```python
from build123d import *

# Parameters (mm, degrees)
SKETCH1_R           = 1.5
BOSS_EXTRUDE1_DEPTH = 38
SKETCH2_R           = 3
BOSS_EXTRUDE2_DEPTH = 8
BOSS_EXTRUDE3_START = -50
SKETCH2_2_R         = 3
BOSS_EXTRUDE3_DEPTH = 8
CHAMFER1_SIZE       = 0.5
SKETCH3_R           = 5
BOSS_EXTRUDE4_DEPTH = 8
CUT_EXTRUDE1_DEPTH  = 8
SKETCH5_R           = 2
CUT_EXTRUDE2_DEPTH  = 47.957427527
CHAMFER3_SIZE       = 1
FILLET1_R           = 2
CHAMFER4_SIZE       = 1


with BuildPart() as part:
    # Sketch1 → Boss-Extrude1 (new, symmetric)
    with BuildSketch(Plane(origin=(0, 0, 0), x_dir=(0, 0, -1), z_dir=(1, 0, 0))):
        Circle(SKETCH1_R)
    extrude(amount=BOSS_EXTRUDE1_DEPTH, both=True)

    # Sketch2 → Boss-Extrude2 (add)
    with BuildSketch(Plane(origin=(38, 0, 0), x_dir=(0, 0, -1), z_dir=(1, 0, 0))):
        Circle(SKETCH2_R)
    extrude(amount=BOSS_EXTRUDE2_DEPTH)

    # Sketch2<2> → Boss-Extrude3 (add)
    with BuildSketch(Plane(origin=(38, 0, 0), x_dir=(0, 0, -1), z_dir=(1, 0, 0)).offset(BOSS_EXTRUDE3_START)):
        Circle(SKETCH2_2_R)
    extrude(amount=BOSS_EXTRUDE3_DEPTH)

    # Chamfer1
    chamfer1_edges = [part.edges().sort_by_distance(p)[0] for p in [
        (-12, 0, 3),
        (-4, 0, 3),
        (38, 0, 3),
        (46, 0, 3),
    ]]
    chamfer(chamfer1_edges, length=CHAMFER1_SIZE)

    # Sketch3 → Boss-Extrude4 (add)
    with BuildSketch(Plane.ZY.offset(38)):
        Circle(SKETCH3_R)
    extrude(amount=-BOSS_EXTRUDE4_DEPTH)

    # Sketch4 → Cut-Extrude1 (cut)
    with BuildSketch(Plane.ZY.offset(38)):
        with BuildLine():
            Line((-4, 3), (-4, -3))
            ThreePointArc((-4, -3), (-5, 0), (-4, 3))
        make_face()
        with BuildLine():
            Line((4, 3), (4, -3))
            ThreePointArc((4, -3), (5, 0), (4, 3))
        make_face()
    extrude(amount=-CUT_EXTRUDE1_DEPTH, mode=Mode.SUBTRACT)

    # Sketch5 → Cut-Extrude2 (cut, through all)
    with BuildSketch(Plane.XY.offset(4)):
        with Locations((-34, 0)):
            Circle(SKETCH5_R)
    extrude(amount=-CUT_EXTRUDE2_DEPTH, mode=Mode.SUBTRACT)

    # Chamfer3
    chamfer3_edges = [part.edges().sort_by_distance(p)[0] for p in [
        (-38, 5, 0),
        (-38, -5, 0),
    ]]
    chamfer(chamfer3_edges, length=CHAMFER3_SIZE - 0.0001)  # a hair under: the kernel refuses the full size

    # Fillet1
    fillet1_edges = [part.edges().sort_by_distance(p)[0] for p in [
        (-30, 0, 1.5),
    ]]
    fillet(fillet1_edges, radius=FILLET1_R)

    # Chamfer4
    chamfer4_edges = [part.edges().sort_by_distance(p)[0] for p in [
        (-30, 5, 0),
        (-30, -5, 0),
    ]]
    chamfer(chamfer4_edges, length=CHAMFER4_SIZE - 0.0001)  # a hair under: the kernel refuses the full size


solid = part.part
```
Geometry: final body of the model. Coordinates: model frame, mm. A direction names the side the tool comes from. Round coordinates to 2 decimals unless told otherwise and drop trailing zeros. Order: outer loops, then holes, each group sorted by start corner. A loop starts at its lowest first (then second) coordinate and runs counter-clockwise, first axis right, second up. Notation, with made-up numbers: (33, 44) -> (38, 44) arc R29 ccw to (38, 74) -> close; hole circle Ø9 at (-8, 30). An arc over 180 degrees is marked (long way). Use one line per item in the form item = value. Start each with the question number.
1. Cut plane C-C (x = 25.5). Return the cut outline in (y, z), then the cut area to 3 significant figures.
2. Cut plane A-A (x = -34). Return the cut outline in (y, z), then the cut area to 3 significant figures.
3. Reachability of faces 4 (the face through (-19.89, 0.07, 1.5)), 5 (the face through (-8, 0, 3)), 6 (the face through (46, 0, 0)) from +Z, -Z, +X, -X, +Y, -Y: full face, straight path, thin tool, end or side. Return the list, or none.
4. Line query: probe 1 along Y at (x, z) = (-34, 1.75); probe 2 along Y at (x, z) = (-34, 2); probe 3 along X at (y, z) = (-2.5, 2.25). Output: solid intervals per line, ascending.
5. Draft query along X for faces 1 (the face through (-30.2, 4.2, 0.1)), 2 (the face through (-34, -5, 0)), 3 (the face through (38, -2, 0)). Return one class per face: pulls with the +X half, pulls with the -X half, needs draft (parallel to the pull), parting line crosses it, or undercut.
6. Pin query (flat end, axial travel): pin 1 Ø6 at (x, y) = (30.5, 0) entering from -Z; pin 2 Ø3 at (x, z) = (-18, 1.5) entering from -Y; pin 3 Ø4 at (x, z) = (23.5, 3) entering from +Y. Return the tip coordinate at first contact, or that it passes through.
7. Cut plane B-B (x = -6). Return the cut outline in (y, z).
Solution:
q1.outline = circle Ø3 at (0, 0)
q1.area = 7.07 mm^2
q2.outline = (-3, -4) -> (-2, -4) -> (-2, 4) -> (-3, 4) arc R5 ccw to start; (2, -4) -> (3, -4) arc R5 ccw to (3, 4) -> (2, 4) -> close
q2.area = 38.4 mm^2
q3.face_4 = none
q3.face_5 = +X
q3.face_6 = +Z, -Z, +X, +Y, -Y
q4.probe_1 = -4.68 to -2, 2 to 4.68
q4.probe_2 = -4.58 to -2, 2 to 4.58
q4.probe_3 = -38 to -30
q5.face_1 = pulls with the +X half
q5.face_2 = needs draft
q5.face_3 = undercut
q6.pin_1 = -1.5
q6.pin_2 = -1.5
q6.pin_3 = 1.12
q7.outline = circle Ø6 at (0, 0)
